Geometry check sheet. Reference: the model listing, model coordinates, mm. A direction names the side the tool comes from. Give positions to 0.01 mm unless a question says otherwise; leave off trailing zeros. Loops run counter-clockwise (first coordinate to the right, second up) from the corner with the lowest first, then second, coordinate; pieces in that order, holes last. Notation, with made-up numbers: (84, 17.5) -> (111, 17.5) arc R28 cw to (111, 53.5) -> close; hole circle Ø3 at (88, 51). An arc over 180 degrees is marked (long way). One line per item, written item: value. Start each with the question number.
(1) Gauge pin test, flat ends, axial feed: pin 1 Ø1.5 at (y, z) = (-117, 121) entering from +X; pin 2 Ø8 at (y, z) = (-231.5, 100) entering from -X; pin 3 Ø12 at (x, z) = (-102, 102.5) entering from -Y. Record the tip position at first contact, or that the pin passes through.
(2) Sectioned sample at A-A, the plane x = 0. Record the cut outline in (y, z).
(3) Tool access check on faces 1 (the face through (-113, 224, 150)), 2 (the face through (-39.054, 297.447, 24.65)), 3 (the face through (4.336, -19.524, 9.86)). Record the directions out of +Z, -Z, +X, -X, +Y, -Y that give a thin tool (end or side, any length) a straight path to the whole face; none if there is none.
(4) Scan lines: line 1 along Y through (x, z) = (0, 5.75); line 2 along Z through (x, y) = (110, 275); line 3 along Y through (x, z) = (-179.5, 9.5). Record each from-to range of solid material in increasing order. Write a range as from..to.
(5) Sectioned sample at D-D, the plane z = 116. Record the cut outline in (x, y).
(6) Sectioned sample at B-B, the plane y = 263.5. Record the cut outline in (x, z).
(7) Draft check along Y on faces 4 (the face through (-4, 4, 200)), 5 (the face through (-39.054, 297.447, 174.65)), 6 (the face through (0, 0, 20)). Enter one of: pulls with the +Y half, pulls with the -Y half, needs draft (parallel to the pull), parting line crosses it, or undercut.
from build123d import *

# Parameters (mm, degrees)
SKETCH1_R           = 300
BOSS_EXTRUDE1_DEPTH = 50
SKETCH2_R           = 20
CUT_EXTRUDE1_DEPTH  = 20
SKETCH4_R           = 250
BOSS_EXTRUDE2_DEPTH = 100
SKETCH6_R           = 300
BOSS_EXTRUDE3_DEPTH = 50


with BuildPart() as part:
    # Sketch1 → Boss-Extrude1 (new body)
    with BuildSketch(Plane.XY):
        Circle(SKETCH1_R)
    extrude(amount=BOSS_EXTRUDE1_DEPTH)

    # Sketch2 → Cut-Extrude1 (cut)
    with BuildSketch(Plane(origin=(0, 0, 0), x_dir=(-1, 0, 0), z_dir=(0, 0, -1))):
        Circle(SKETCH2_R)
    extrude(amount=-CUT_EXTRUDE1_DEPTH, mode=Mode.SUBTRACT)

    # Sketch4 → Boss-Extrude2 (add)
    with BuildSketch(Plane.XY.offset(50)):
        Circle(SKETCH4_R)
    extrude(amount=BOSS_EXTRUDE2_DEPTH)

    # Sketch6 → Boss-Extrude3 (add)
    with BuildSketch(Plane.XY.offset(150)):
        Circle(SKETCH6_R)
    extrude(amount=BOSS_EXTRUDE3_DEPTH)


solid = part.part
Calculated:
1. pin 1: stops at x = 221.33
1. pin 2: stops at x = -103.65
1. pin 3: stops at y = -230.83
2. outline: (-300, 0) -> (-20, 0) -> (-20, 20) -> (20, 20) -> (20, 0) -> (300, 0) -> (300, 50) -> (250, 50) -> (250, 150) -> (300, 150) -> (300, 200) -> (-300, 200) -> (-300, 150) -> (-250, 150) -> (-250, 50) -> (-300, 50) -> close
3. face 1: none
3. face 2: +Z, -Z
3. face 3: -Z
4. line 1: y = -300..-20, 20..300
4. line 2: z = 0..50, 150..200
4. line 3: y = -240.37..240.37
5. outline: circle Ø500 at (0, 0)
6. outline: (-143.41, 0) -> (143.41, 0) -> (143.41, 50) -> (-143.41, 50) -> close; (-143.41, 150) -> (143.41, 150) -> (143.41, 200) -> (-143.41, 200) -> close
7. face 4: needs draft
7. face 5: parting line crosses it
7. face 6: undercut
